Verification items for the finished model (mm, model axes). Face numbers are marked on the shaded views. A direction names the side the tool comes from. Round coordinates to 2 decimals unless told otherwise and drop trailing zeros. Write each loop counter-clockwise with the first axis right and the second up, starting at its lowest first coordinate (ties: lowest second). Pieces come first, ordered by that corner, then holes. Notation, with made-up numbers: (50.25, 82) - (92.25, 82) arc R10 cw to (92.25, 90) - close; hole circle Ø1 at (9, -35.5). An arc over 180 degrees is marked (long way). Answer as a JSON object with one key per item and string values.
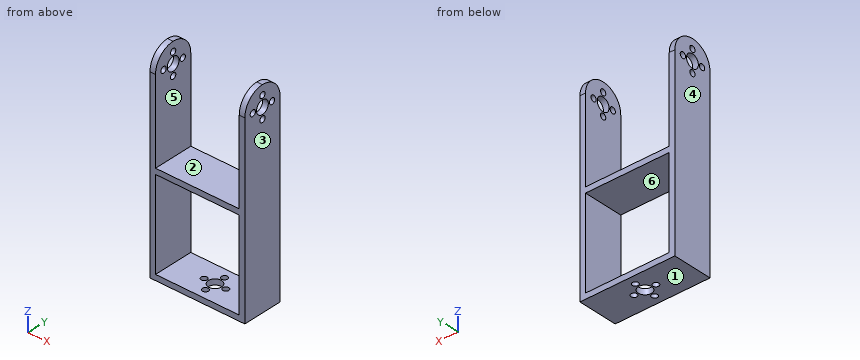
```python
from build123d import *

# Parameters (mm, degrees)
F0_W      = 60.325
F0_H      = 25.4
F1_DEPTH  = 3.556
F2_W      = 3.556
F2_H      = 25.4
F3_DEPTH  = 127
F4_R      = 12.7
F5_R      = 12.69999
F6_R      = 4.2545
F6_R_2    = 1.905
F7_DEPTH  = 254
F8_R      = 4.2545
F8_R_2    = 1.905
F9_DEPTH  = 25.4
F10_W     = 25.4
F10_H     = 3.556
F11_DEPTH = 53.34


# Not quite as in the source:
# - a fillet or chamfer is up to 0.001 mm smaller than in the source, because OpenCascade refuses the exact size


with BuildPart() as f1:
    # F0 (on Top) → F1 (new body)
    with BuildSketch(Plane.XY):
        with Locations((3.8735, 0)):
            Rectangle(F0_W, F0_H)
    extrude(amount=F1_DEPTH)

    # F2 (on face) → F3 (join)
    with BuildSketch(Plane.XY.offset(3.556)):
        with Locations((-24.511, 0)):
            Rectangle(F2_W, F2_H)
        with Locations((32.258, 0)):
            Rectangle(F2_W, F2_H)
    extrude(amount=F3_DEPTH)

    # F4
    f4_edges = [f1.edges().sort_by_distance(p)[0] for p in [
        (32.258, 12.7, 130.556),
    ]]
    fillet(f4_edges, radius=F4_R)

    # F5 (radius 12.7 in the source; OpenCascade refuses exactly that, so slightly less here)
    f5_edges = [f1.edges().sort_by_distance(p)[0] for p in [
        (32.258, -12.7, 130.556),
        (-24.511, -12.7, 130.556),
        (-24.511, 12.7, 130.556),
    ]]
    fillet(f5_edges, radius=F5_R)

    # F6 (on face) → F7 (cut)
    with BuildSketch(Plane.YZ.offset(34.036)):
        with Locations((0, 117.6655)):
            Circle(F6_R)
        with Locations((0, 124.587)):
            Circle(F6_R_2)
        with Locations((-6.9215, 117.6655)):
            Circle(F6_R_2)
        with Locations((0, 110.744)):
            Circle(F6_R_2)
        with Locations((6.9215, 117.6655)):
            Circle(F6_R_2)
    extrude(amount=-F7_DEPTH, mode=Mode.SUBTRACT)

    # F8 (on face) → F9 (cut)
    with BuildSketch(Plane.XY.offset(3.556)):
        with Locations((3.8735, 0)):
            Circle(F8_R)
        with Locations((-3.048, 0)):
            Circle(F8_R_2)
        with Locations((3.8735, 6.9215)):
            Circle(F8_R_2)
        with Locations((3.8735, -6.9215)):
            Circle(F8_R_2)
        with Locations((10.795, 0)):
            Circle(F8_R_2)
    extrude(amount=-F9_DEPTH, mode=Mode.SUBTRACT)

    # F10 (on face) → F11 (join)
    with BuildSketch(Plane.YZ.offset(-22.733)):
        with Locations((0, 62.484)):
            Rectangle(F10_W, F10_H)
    extrude(amount=F11_DEPTH)


solid = f1.part
```
Q1. Set-up check for the marked faces 4, 5 and 6: record each of +Z, -Z, +X, -X, +Y, -Y from which the full face is reachable in a straight line by a thin tool's end or side.
Geometry check:
{"face 4": "+Z, -Z, -X, +Y, -Y", "face 5": "+Z, +Y, -Y", "face 6": "+Y, -Y"}
Q2. Gauge pin test, flat ends, axial feed: P1, Ø3.5, axis at y = 0, z = 110.744, coming from the -X side; P2, Ø3, axis at x = 3.87, y = -6.92, coming from the -Z side; P3, Ø2.5, axis at x = 3.87, y = 6.92, coming from the +Z side. Record the tip position at first contact, or that the pin passes through.
Geometry check:
{"P1": "passes through", "P2": "stops at z = 60.71", "P3": "stops at z = 64.26"}
Q3. Release check for a two-part mould opening along X. For the marked faces 1, 2 and 3 record: released by +X, released by -X, zero draft, split by the parting line, or undercut.
Geometry check:
{"face 1": "zero draft", "face 2": "undercut", "face 3": "released by +X"}
Q4. Section check A-A, the plane z = 104.5. Record the cut outline in (x, y), then the cut area to 3 significant figures.
Geometry check:
{"outline": "(-26.29, -12.7) - (-22.73, -12.7) - (-22.73, 12.7) - (-26.29, 12.7) - close; (30.48, -12.7) - (34.04, -12.7) - (34.04, 12.7) - (30.48, 12.7) - close", "area": "181 mm2"}
Q5. Material ranges on line 1 along X through (y, z) = (7.75, 103); line 2 along Z through (x, y) = (-6, -10.5), recorded low to high. Write a range as [from, to].
Geometry check:
{"line 1": "x = [-26.29, -22.73], [30.48, 34.04]", "line 2": "z = [0, 3.56], [60.71, 64.26]"}
